Geometry check sheet. Reference: the model listing, model coordinates, mm. A direction names the side the tool comes from. Coordinates: 2 decimals unless noted, no trailing zeros. Loops run counter-clockwise (first coordinate to the right, second up) from the corner with the lowest first, then second, coordinate; pieces in that order, holes last. Notation, with made-up numbers: M 77.5,34.5 L 83.5,34.5 A23 ccw 83.5,67.5 Z; hole C 62.5,59.25 d10. An arc over 180 degrees is marked long. Use CSV: the item, a comma, the result in double quotes.
```python
from build123d import *

# Parameters (mm, degrees)
SKETCH1_W           = 25.4
SKETCH1_H           = 50.8
SKETCH1_W_2         = 22.225
SKETCH1_H_2         = 47.625
BOSS_EXTRUDE1_DEPTH = 838.2
SKETCH2_R           = 3.175
CUT_EXTRUDE1_DEPTH  = 839.969343898
CUT_EXTRUDE2_REACH  = 840.969
SKETCH3_R           = 6.35


with BuildPart() as part:
    # Sketch1 → Boss-Extrude1 (new body)
    with BuildSketch(Plane.XY):
        Rectangle(SKETCH1_W, SKETCH1_H)
        Rectangle(SKETCH1_W_2, SKETCH1_H_2, mode=Mode.SUBTRACT)
    extrude(amount=BOSS_EXTRUDE1_DEPTH)

    # Sketch2 → Cut-Extrude1 (cut, through all)
    with BuildSketch(Plane(origin=(12.7, 0, 0), x_dir=(0, 0, -1), z_dir=(1, 0, 0))):
        with Locations((-85.725, 12.7)):
            Circle(SKETCH2_R)
        with Locations((-85.725, -12.7)):
            Circle(SKETCH2_R)
        with Locations((-752.475, 12.7)):
            Circle(SKETCH2_R)
        with Locations((-752.475, -12.7)):
            Circle(SKETCH2_R)
    extrude(amount=-CUT_EXTRUDE1_DEPTH, mode=Mode.SUBTRACT)

    # Sketch3 → Cut-Extrude2 (cut, up to next)
    with BuildSketch(Plane(origin=(12.7, 0, 0), x_dir=(0, 0, -1), z_dir=(1, 0, 0)), mode=Mode.PRIVATE) as cut_extrude2_sk1:
        with Locations((-752.475, 12.7)):
            Circle(SKETCH3_R)
    cut_extrude2_tool1 = extrude(cut_extrude2_sk1.sketch, amount=-CUT_EXTRUDE2_REACH, mode=Mode.PRIVATE) & part.part
    # Sketch3 → Cut-Extrude2 (cut, up to next)
    with BuildSketch(Plane(origin=(12.7, 0, 0), x_dir=(0, 0, -1), z_dir=(1, 0, 0)), mode=Mode.PRIVATE) as cut_extrude2_sk2:
        with Locations((-752.475, -12.7)):
            Circle(SKETCH3_R)
    cut_extrude2_tool2 = extrude(cut_extrude2_sk2.sketch, amount=-CUT_EXTRUDE2_REACH, mode=Mode.PRIVATE) & part.part
    # Sketch3 → Cut-Extrude2 (cut, up to next)
    with BuildSketch(Plane(origin=(12.7, 0, 0), x_dir=(0, 0, -1), z_dir=(1, 0, 0)), mode=Mode.PRIVATE) as cut_extrude2_sk3:
        with Locations((-85.725, 12.7)):
            Circle(SKETCH3_R)
    cut_extrude2_tool3 = extrude(cut_extrude2_sk3.sketch, amount=-CUT_EXTRUDE2_REACH, mode=Mode.PRIVATE) & part.part
    # Sketch3 → Cut-Extrude2 (cut, up to next)
    with BuildSketch(Plane(origin=(12.7, 0, 0), x_dir=(0, 0, -1), z_dir=(1, 0, 0)), mode=Mode.PRIVATE) as cut_extrude2_sk4:
        with Locations((-85.725, -12.7)):
            Circle(SKETCH3_R)
    cut_extrude2_tool4 = extrude(cut_extrude2_sk4.sketch, amount=-CUT_EXTRUDE2_REACH, mode=Mode.PRIVATE) & part.part
    add(cut_extrude2_tool1.solids().sort_by_distance((12.7, 12.7, 752.475))[0], mode=Mode.SUBTRACT)
    add(cut_extrude2_tool2.solids().sort_by_distance((12.7, -12.7, 752.475))[0], mode=Mode.SUBTRACT)
    add(cut_extrude2_tool3.solids().sort_by_distance((12.7, 12.7, 85.725))[0], mode=Mode.SUBTRACT)
    add(cut_extrude2_tool4.solids().sort_by_distance((12.7, -12.7, 85.725))[0], mode=Mode.SUBTRACT)


solid = part.part
```
1. Release check for a two-part mould opening along Y. For faces 1 (the flat face through (0, -25.4, 413)), 2 (the flat face through (-11.3, 2, 838.2)), 3 (the flat face through (11.112, 0, 413)) record: +Y half, -Y half, draft (parallel to the pull), parting line (faces both ways), or undercut.
The answers:
face 1,"-Y half"
face 2,"draft"
face 3,"undercut"
2. Section check B-B, the plane x = -0.5. Record the cut outline in (y, z), plus the area to 3 significant figures.
The answers:
outline,"M -25.4,0 L -23.81,0 L -23.81,838.2 L -25.4,838.2 Z; M 23.81,0 L 25.4,0 L 25.4,838.2 L 23.81,838.2 Z"
area,"2,660 mm^2"
3. Set-up check for faces 4 (the flat face through (0, 25.4, 413)), 5 (the flat face through (0, -23.812, 413)), 6 (the cylindrical face through (11.9, 17, 90.4)): record each of +Z, -Z, +X, -X, +Y, -Y from which the full face is reachable in a straight line by a thin tool's end or side.
The answers:
face 4,"+Z, -Z, +X, -X, +Y"
face 5,"+Z, -Z"
face 6,"+X"
4. Section check A-A, the plane z = 236. Record the cut outline in (x, y).
The answers:
outline,"M -12.7,-25.4 L 12.7,-25.4 L 12.7,25.4 L -12.7,25.4 Z; hole M -11.11,-23.81 L 11.11,-23.81 L 11.11,23.81 L -11.11,23.81 Z"
5. Gauge pin test, flat ends, axial feed: P1, Ø10, axis at y = 12.7, z = 752.475, coming from the +X side; P2, Ø5.5, axis at y = 12.7, z = 85.725, coming from the +X side. Record the tip position at first contact, or that the pin passes through.
The answers:
P1,"x = -11.11"
P2,"through"
6. Thickness scan on line 1 (X direction, y = 1, z = 726); line 2 (Y direction, x = 10.25, z = 457). Record the ranges inside material, lowest first. Write a range as [from, to].
The answers:
line 1,"[-12.7, -11.11], [11.11, 12.7]"
line 2,"[-25.4, -23.81], [23.81, 25.4]"
